```python
from build123d import *

# Parameters (mm, degrees)
F0_W     = 800
F0_H     = 1500
F1_DEPTH = 25
F2_R     = 25
F3_DEPTH = 700
F6_R     = 100


with BuildPart() as f1:
    # F0 (on Top) → F1 (new body)
    with BuildSketch(Plane.XY):
        Rectangle(F0_W, F0_H)
    extrude(amount=F1_DEPTH)

    # F2 (on face) → F3 (join)
    with BuildSketch(Plane.XY.offset(25)):
        with Locations((-275, 625)):
            Circle(F2_R)
    extrude(amount=F3_DEPTH)

    # F4: F1 across plane


with BuildPart() as f1_1:
    add(f1.part)
    add(f1.part.mirror(Plane.XZ))

    # F5: F1 across plane


with BuildPart() as f1_2:
    add(f1_1.part)
    add(f1_1.part.mirror(Plane.YZ))

    # F6
    f6_edges = [f1_2.edges().sort_by_distance(p)[0] for p in [
        (-400, 750, 12.5),
        (400, 750, 12.5),
        (400, -750, 12.5),
        (-400, -750, 12.5),
    ]]
    fillet(f6_edges, radius=F6_R)


solid = f1_2.part
```
Can you work these out from the model? Positions are in its coordinate system, mm. A direction names the side the tool comes from. Coordinates: 2 decimals unless noted, no trailing zeros. Loops run counter-clockwise (first coordinate to the right, second up) from the corner with the lowest first, then second, coordinate; pieces in that order, holes last. Notation, with made-up numbers: (-39, 75) -> (14, 75) arc R16 cw to (14, 101) -> close; hole circle Ø4 at (-3.5, 8.5). An arc over 180 degrees is marked (long way). Put each result on its own line as item: value. Start each with the question number.
Q1. I want a section at D-D (y = 63). Write out the boundary of the cut face in (x, z), plus the area to 3 significant figures.
Q2. Thinking about a two-plate mould opening in X: for faces 3 (the face through (369.929, -721.484, 12.675)), 4 (the face through (263.5, 602.8, 370.1)), 5 (the face through (-263.5, 602.8, 370.1)), 6 (the face through (-371.484, 719.929, 12.675)), which applies, pulls with the +X half, pulls with the -X half, needs draft (parallel to the pull), parting line crosses it, or undercut?
Q3. I want a section at A-A (x = 275). Write out the boundary of the cut face in (y, z).
Q4. I want a section at B-B (z = 162). Write out the boundary of the cut face in (x, y), plus the area to 3 significant figures.
Q5. For faces 1 (the face through (-275, -625, 725)), 2 (the face through (-263.5, -602.8, 370.1)), which set-ups out of +Z, -Z, +X, -X, +Y, -Y let a thin tool reach every point of the face, with its end or its side?
Q6. I'm going to push flat-ended pins straight in: P1, Ø10, axis at x = 86.5, y = 529, coming from the +Z side; P2, Ø1, axis at x = 288.5, z = 150.5, coming from the +Y side. Where does each tip first touch, or does it pass through?
Q7. I want a section at C-C (y = 625). Write out the boundary of the cut face in (x, z).
Q8. If I drill on line 1 (Z direction, x = -77.5, y = -363); line 2 (Y direction, x = -257, z = 602); line 3 (X direction, y = -627.5, z = 119.5), over which ranges is the centre line in solid material (lowest first)? Write a range as [from, to].
Taken from the geometry:
1. outline: (-400, 0) -> (400, 0) -> (400, 25) -> (-400, 25) -> close
1. area: 20,000 mm2
2. face 3: pulls with the +X half
2. face 4: undercut
2. face 5: undercut
2. face 6: pulls with the -X half
3. outline: (-750, 0) -> (750, 0) -> (750, 25) -> (650, 25) -> (650, 725) -> (600, 725) -> (600, 25) -> (-600, 25) -> (-600, 725) -> (-650, 725) -> (-650, 25) -> (-750, 25) -> close
4. outline: circle Ø50 at (-275, -625); circle Ø50 at (-275, 625); circle Ø50 at (275, -625); circle Ø50 at (275, 625)
4. area: 7,850 mm2
5. face 1: +Z, +X, -X, +Y, -Y
5. face 2: +Z
6. P1: stops at z = 25
6. P2: stops at y = 646.35
7. outline: (-400, 0) -> (400, 0) -> (400, 25) -> (300, 25) -> (300, 725) -> (250, 725) -> (250, 25) -> (-250, 25) -> (-250, 725) -> (-300, 725) -> (-300, 25) -> (-400, 25) -> close
8. line 1: z = [0, 25]
8. line 2: y = [-642.35, -607.65], [607.65, 642.35]
8. line 3: x = [-299.87, -250.13], [250.13, 299.87]
